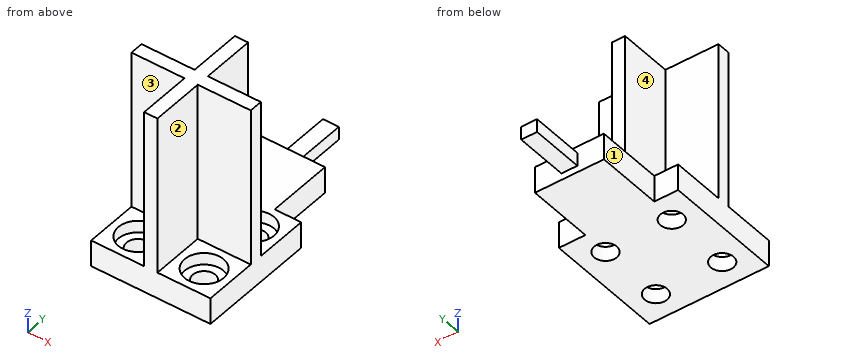
Autodesk Fusion 360 part; units mm, degrees
sketch "Sketch1" plane through (0, 0, 0) normal (0, 0, 1) x (1, 0, 0)
  line L0 (-1, 10) -> (5, 10)
  line L1 (5, 10) -> (5, -10)
  line L2 (5, -10) -> (-1, -10)
  line L3 (-1, -10) -> (-1, 10)
  line L4 (-1, -10) -> (-11, -10)
  line L5 (5, -10) -> (15, -10)
  line L6 (-11, -10) -> (-11, -35)
  line L7 (15, -10) -> (15, -35)
  line L8 (-11, -35) -> (-20, -35)
  line L9 (-20, -35) -> (-20, -80)
  line L10 (15, -35) -> (25, -35)
  line L11 (-20, -80) -> (25, -80)
  line L12 (25, -80) -> (25, -35)
  dimension "d1" = 20
  dimension "d2" = 10
  dimension "d3" = 6
  dimension "d4" = 10
  dimension "d5" = 45
extrude "Extrude1" add sketch "Sketch1" along normal blind 5 contours L0 L1 L2 L3
sketch "Sketch2" plane through (0, 0, 5) normal (0, 0, 1) x (-1, 0, 0)
  line L0 (-5, 10) -> (-5, -10)
  line L1 (-5, -10) -> (1, -10)
  line L2 (1, -10) -> (1, 10)
  line L3 (-25, 55) -> (-25, 60)
  line L4 (-25, 60) -> (20, 60)
  line L5 (20, 55) -> (-25, 55)
  line L6 (-2.5, 35) -> (-5, 35)
  line L7 (-5, 35) -> (-5, 80)
  line L8 (-2.5, 35) -> (0, 35)
  line L9 (0, 35) -> (0, 80)
  line L10 (1, 10) -> (-5, 10)
  line L11 (-5, 80) -> (-2.5, 80)
  line L12 (0, 80) -> (-2.5, 80)
  line L13 (20, 60) -> (19.7373, 60)
  line L14 (20, 55) -> (20, 57.5)
  line L15 (20, 60) -> (20, 57.5)
extrude "Extrude2" add sketch "Sketch1" along normal blind 7.5 contours L2 L4 L5 L6 L7 L8 L9 L10 L11 L12
extrude "Extrude3" add sketch "Sketch1" against normal blind 2.5 contours L2 L4 L5 L6 L7 L8 L9 L10 L11 L12
extrude "Extrude4" add sketch "Sketch2" along normal blind 62.6 contours L3 L4 L5 L7 | L4 L5 L7 L9 | L5 L6 L7 L8 L9 | L4 L7 L9 L11 L12 | L4 L5 L9 L13 L14 L15
sketch "Sketch3" plane through (0, 0, 7.5) normal (0, 0, 1) x (-1, 0, 0)
  line L0 (20, 55) -> (0, 55)
  line L1 (0, 55) -> (0, 35)
  line L2 (0, 35) -> (-5, 35)
  line L3 (-5, 35) -> (-5, 55)
  line L4 (-5, 55) -> (-25, 55)
  line L5 (-25, 55) -> (-25, 35)
  line L6 (-25, 35) -> (-15, 35)
  line L7 (-15, 35) -> (-15, 10)
  line L8 (-15, 10) -> (11, 10)
  line L9 (11, 10) -> (11, 35)
  line L10 (11, 35) -> (20, 35)
  line L11 (20, 35) -> (20, 55)
  circle A0 centre (-15, 45) radius 7.35
  circle A1 centre (-15, 70) radius 7.35
  circle A2 centre (10, 70) radius 7.35
  circle A3 centre (10, 45) radius 7.35
  line L12 (0, 80) -> (0, 60)
  line L13 (0, 60) -> (20, 60)
  line L14 (-5, 60) -> (-5, 80)
  line L15 (-25, 60) -> (-5, 60)
  dimension "d15" = 10
  dimension "d16" = 10
  dimension "d17" = 10
  dimension "d18" = 10
  dimension "d19" = 10
  dimension "d20" = 10
  dimension "d21" = 10
  dimension "d22" = 10
  dimension "d23" = 14.7
  dimension "d24" = 14.7
  dimension "d25" = 14.7
  dimension "d26" = 14.7
extrude "Extrude5" cut sketch "Sketch3" against normal blind 4.5 contours A0 | A1 | A2 | A3
sketch "Sketch4" plane through (0, 0, 3) normal (0, 0, 1) x (-1, 0, 0)
  circle A0 centre (-15, 45) radius 7.35
  circle A1 centre (-15, 70) radius 4.25
  circle A2 centre (10, 70) radius 4.25
  circle A3 centre (10, 45) radius 4.25
  circle A4 centre (-15, 45) radius 4.25
  line L0 (0, 60) -> (20, 60)
  dimension "d29" = 10
  dimension "d30" = 8.5
  dimension "d31" = 8.5
  dimension "d32" = 8.5
  dimension "d33" = 8.5
extrude "Extrude6" cut sketch "Sketch4" against normal blind 6 contours A1 | A2 | A3 | A4
Verification items for the finished model (mm, model axes). Face numbers are marked on the shaded views. A direction names the side the tool comes from. Give positions to 0.01 mm unless a question says otherwise; leave off trailing zeros. Order: outer loops, then holes, each group sorted by start corner. A loop starts at its lowest first (then second) coordinate and runs counter-clockwise, first axis right, second up. Notation, with made-up numbers: M 87.5,-28 L 122.5,-28 A13 cw 122.5,-12 Z; hole C -18,-25.75 d7. An arc over 180 degrees is marked long. Answer in a Markdown table with one row per item. Add a question column.
Item 1: Section check D-D, the plane y = -25.5. Enter the section's corners in (x, z).
Item 2: Section check C-C, the plane z = 21.5. Enter the section's corners in (x, y).
Item 3: Tool access check on the marked faces 1, 2, 3 and 4. Record the directions out of +Z, -Z, +X, -X, +Y, -Y that give a thin tool (end or side, any length) a straight path to the whole face; none if there is none.
Item 4: Scan lines: probe 1 along X at (y, z) = (-45, 0); probe 2 along X at (y, z) = (-70, 6); probe 3 along Z at (x, y) = (-4.5, -68.5). Record each from-to range of solid material in increasing order. Write a range as from..to.
Item 5: Section check A-A, the plane x = -10. Enter the section's corners in (y, z), and give its area (3 significant figures).
Item 6: Gauge pin test, flat ends, axial feed: pin 1 (5 mm diameter, centred on x = 15.5, z = 16, fed in from -Y); pin 2 (8 mm diameter, centred on x = -12.5, z = 59.5, fed in from +Y); pin 3 (1.5 mm diameter, centred on y = -1, z = 2.5, fed in from +X); pin 4 (7 mm diameter, centred on x = 15, y = -45, fed in from +Z). Record the tip position at first contact, or that the pin passes through.
Item 7: Section check B-B, the plane y = -45. Enter the section's corners in (x, z), and give its area (3 significant figures).
Filled sheet:
| question | item | result |
|---|---|---|
| 1 | outline | M -11,-2.5 L 15,-2.5 L 15,7.5 L -11,7.5 Z |
| 2 | outline | M -20,-60 L 0,-60 L 0,-80 L 5,-80 L 5,-60 L 25,-60 L 25,-55 L 5,-55 L 5,-35 L 0,-35 L 0,-55 L -20,-55 Z |
| 3 | face 1 | +Z, -Z, -X, +Y |
| 3 | face 2 | +Z, +X, -Y |
| 3 | face 3 | +Z, -X, -Y |
| 3 | face 4 | +Z, -X, +Y |
| 4 | probe 1 | x = -20..-14.25, -5.75..10.75, 19.25..25 |
| 4 | probe 2 | x = -20..-17.35, -2.65..7.65, 22.35..25 |
| 4 | probe 3 | z = -2.5..3 |
| 5 | outline | M -80,-2.5 L -74.25,-2.5 L -74.25,3 L -77.35,3 L -77.35,7.5 L -80,7.5 Z; M -65.75,-2.5 L -49.25,-2.5 L -49.25,3 L -52.35,3 L -52.35,7.5 L -55,7.5 L -55,67.6 L -60,67.6 L -60,7.5 L -62.65,7.5 L -62.65,3 L -65.75,3 Z; M -40.75,-2.5 L -10,-2.5 L -10,7.5 L -37.65,7.5 L -37.65,3 L -40.75,3 Z |
| 5 | area | 775 mm^2 |
| 6 | pin 1 | stops at y = -60 |
| 6 | pin 2 | stops at y = -55 |
| 6 | pin 3 | stops at x = 5 |
| 6 | pin 4 | passes through |
| 7 | outline | M -20,-2.5 L -14.25,-2.5 L -14.25,3 L -17.35,3 L -17.35,7.5 L -20,7.5 Z; M -5.75,-2.5 L 10.75,-2.5 L 10.75,3 L 7.65,3 L 7.65,7.5 L 5,7.5 L 5,67.6 L 0,67.6 L 0,7.5 L -2.65,7.5 L -2.65,3 L -5.75,3 Z; M 19.25,-2.5 L 25,-2.5 L 25,7.5 L 22.35,7.5 L 22.35,3 L 19.25,3 Z |
| 7 | area | 525 mm^2 |
